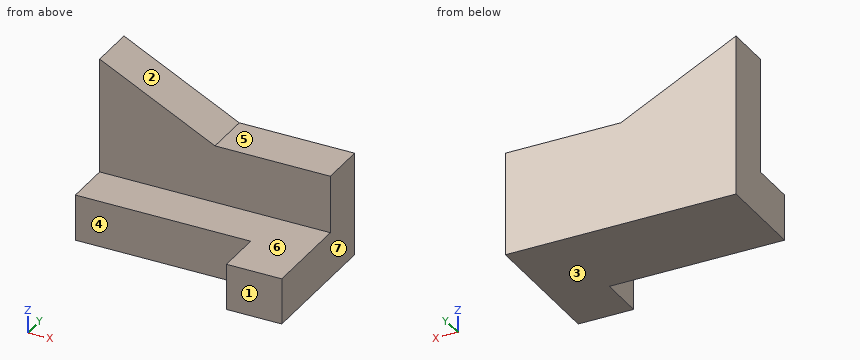
from build123d import *

# Parameters (mm, degrees)
F0_W     = 50
F0_H     = 35
F1_DEPTH = 30
F2_W     = 20
F2_H     = 25
F3_DEPTH = 50.001
F4_W     = 38
F4_H     = 10
F5_DEPTH = 10.001
F7_DEPTH = 10.001


with BuildPart() as f1:
    # F0 (on Front) → F1 (new body)
    with BuildSketch(Plane.XZ):
        with Locations((25, 17.5)):
            Rectangle(F0_W, F0_H)
    extrude(amount=F1_DEPTH)

    # F2 (on face) → F3 (cut, through all)
    with BuildSketch(Plane.YZ.offset(50)):
        with Locations((-20, 22.5)):
            Rectangle(F2_W, F2_H)
    extrude(amount=-F3_DEPTH, mode=Mode.SUBTRACT)

    # F4 (on face) → F5 (cut, through all)
    with BuildSketch(Plane.XY.offset(10)):
        with Locations((19, -25)):
            Rectangle(F4_W, F4_H)
    extrude(amount=-F5_DEPTH, mode=Mode.SUBTRACT)

    # F6 (on face) → F7 (cut, through all)
    with BuildSketch(Plane.XZ.offset(10)):
        Polygon((50, 35), (0, 35), (25, 22.5), (50, 22.5), align=None)
    extrude(amount=-F7_DEPTH, mode=Mode.SUBTRACT)


solid = f1.part
CAD build for the part. Positions are in the model's coordinates, mm. Face numbers are marked on the shaded views. A direction names the side the tool comes from. Round coordinates to 2 decimals unless told otherwise and drop trailing zeros. Order: outer loops, then holes, each group sorted by start corner. A loop starts at its lowest first (then second) coordinate and runs counter-clockwise, first axis right, second up. Notation, with made-up numbers: M -17,-8 L 1,-8 A17 ccw 1,9 Z; hole C -12.5,32.5 d9. An arc over 180 degrees is marked long. Use one line per item in the form item = value.
Q1. Which spindle directions (+Z, -Z, +X, -X, +Y, -Y) get a long thin tool onto all of the face, cutting with end or side? Do the marked faces 4, 5, 6 and 7. Say none if no direction does.
Recorded:
face_4 = +Z, -Z, -X, -Y
face_5 = +Z, +X, +Y, -Y
face_6 = +Z, +X, -X, -Y
face_7 = +Z, -Z, +X, +Y, -Y
Q2. Probe L1, parallel to Z at x = 43, y = -8; L2, parallel to Y at x = 46.5, z = 15; L3, parallel to Y at x = 7, z = 9. List the from-to ranges inside material, lowest first.
Recorded:
L1 = 0 to 22.5
L2 = -10 to 0
L3 = -20 to 0
Q3. Two-plate mould, pull along Z, no slides. Class the marked faces 1, 2 and 3: +Z half, -Z half, draft (parallel to the pull), parting line (faces both ways), or undercut.
Recorded:
face_1 = draft
face_2 = +Z half
face_3 = -Z half
Q4. Saw through at B-B on x = 11.5. Give the cut face in (y, z).
Recorded:
outline = M -20,0 L 0,0 L 0,29.25 L -10,29.25 L -10,10 L -20,10 Z
Q5. Saw through at C-C on y = -7. Give the cut face in (x, z), then the cut area to 3 significant figures.
Recorded:
outline = M 0,0 L 50,0 L 50,22.5 L 25,22.5 L 0,35 Z
area = 1,280 mm^2
Q6. Flat gauge pins, fed straight in: P1, Ø4, axis at x = 20, z = 16, coming from the -Y side; P2, Ø6, axis at x = 24, y = -24.5, coming from the +Z side; P3, Ø8, axis at x = 35, y = -7.5, coming from the +Z side; P4, Ø12, axis at x = 9, y = -17.5, coming from the +Z side. Where does each tip first touch, or does it go through?
Recorded:
P1 = -10
P2 = through
P3 = 22.5
P4 = 10
Q7. Saw through at A-A on z = 9. Give the cut face in (x, y).
Recorded:
outline = M 0,-20 L 38,-20 L 38,-30 L 50,-30 L 50,0 L 0,0 Z
Q8. Saw through at D-D on z = 30.5. Give the cut face in (x, y), then the cut area to 3 significant figures.
Recorded:
outline = M 0,-10 L 9,-10 L 9,0 L 0,0 Z
area = 90.0 mm^2
